Drawing for the job (mm, zero at the part's lowest x, y, z). Give positions to 0.01 mm unless a question says otherwise; leave off trailing zeros. Loops run counter-clockwise (first coordinate to the right, second up) from the corner with the lowest first, then second, coordinate; pieces in that order, holes last. Notation, with made-up numbers: (17, 73) - (62, 73) arc R28 ccw to (62, 98) - close; hole circle Ø8 at (85, 25). An arc over 180 degrees is marked (long way). Return JSON: item names as keys, results as strings. Group by question number.
1) Slice it at C-C (z = 23). List the corners of the cut face in (x, y), and give its area (3 significant figures).
2) Drop flat-ended pins along their axis: pin 1 (5 mm diameter, centred on x = 6, y = 15, fed in from +Z); pin 2 (3 mm diameter, centred on x = 2, y = 51.5, fed in from +Z); pin 3 (5 mm diameter, centred on x = 1.5, z = 53.5, fed in from +Y). Give the stop position or say it passes through.
3) Slice it at A-A (x = 6). List the corners of the cut face in (y, z), and give its area (4 significant figures).
4) Slice it at D-D (z = 60.5). List the corners of the cut face in (x, y), and give its area (3 significant figures).
5) Drill centre lines: probe 1 along X at (y, z) = (15, 14); probe 2 along Y at (x, z) = (3.5, 8); probe 3 along Y at (x, z) = (7, 10.5). Where is each one in solid material? Low to high. Write a range as from..to.
6) Slice it at B-B (y = 15). List the corners of the cut face in (x, z).
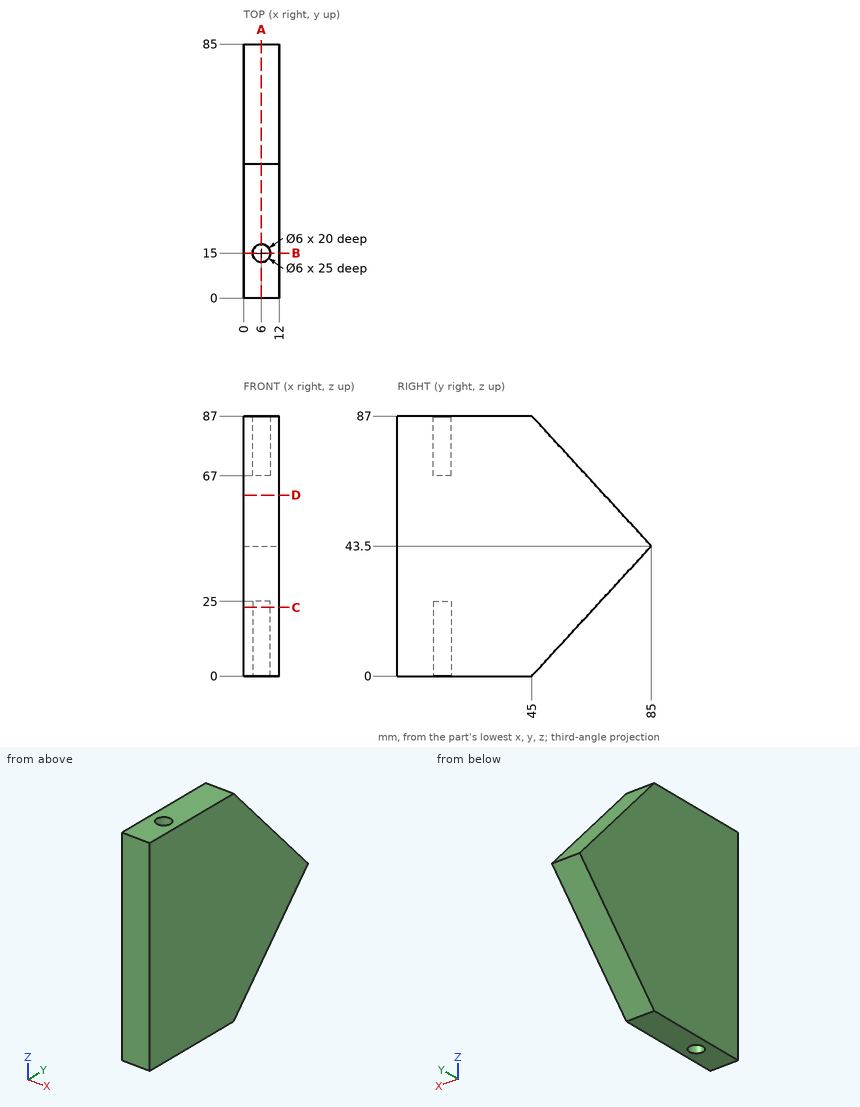
Results:
{
 "1": {"outline": "(0, 0) - (12, 0) - (12, 66.15) - (0, 66.15) - close; hole circle Ø6 at (6, 15)", "area": "766 mm2"},
 "2": {"pin 1": "z = 67", "pin 2": "z = 81.56", "pin 3": "y = 78.1"},
 "3": {"outline": "(0, 0) - (12, 0) - (12, 25) - (18, 25) - (18, 0) - (45, 0) - (85, 43.5) - (45, 87) - (18, 87) - (18, 67) - (12, 67) - (12, 87) - (0, 87) - close", "area": "5,385 mm2"},
 "4": {"outline": "(0, 0) - (12, 0) - (12, 69.37) - (0, 69.37) - close", "area": "832 mm2"},
 "5": {"probe 1": "0..3, 9..12", "probe 2": "0..13.34, 16.66..52.36", "probe 3": "0..12.17, 17.83..54.66"},
 "6": {"outline": "(0, 0) - (3, 0) - (3, 25) - (9, 25) - (9, 0) - (12, 0) - (12, 87) - (9, 87) - (9, 67) - (3, 67) - (3, 87) - (0, 87) - close"}
}
